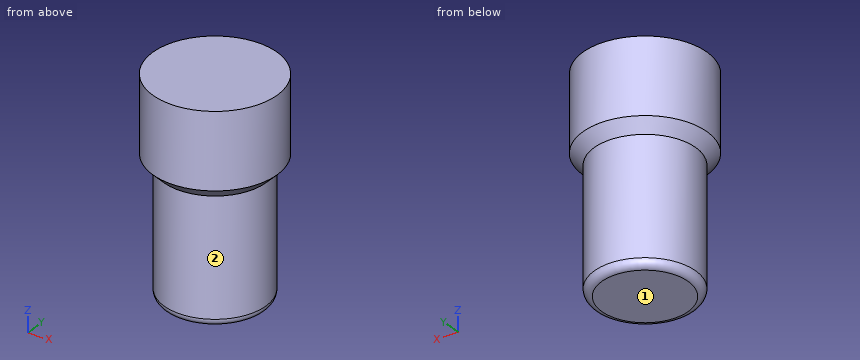
Autodesk Inventor part; units mm, degrees
ref_plane "YZ Plane" through (0, 0, 0) normal (1, 0, 0) x (0, 1, 0)
ref_plane "XZ Plane" through (0, 0, 0) normal (0, 1, 0) x (-1, 0, 0)
ref_plane "XY Plane" through (0, 0, 0) normal (0, 0, 1) x (1, 0, 0)
sketch "Sketch1" plane through (0, 0, 0) normal (0, 0, 1) x (1, 0, 0)
  circle A0 centre (0, 0) radius 13.5
  dimension "d0" = 27
extrude "Extrusion1" add sketch "Sketch1" along normal blind 36
sketch "Sketch2" plane through (0, 0, 36) normal (0, 0, 1) x (1, 0, 0)
  circle A0 centre (0, 0) radius 16.5
  dimension "d3" = 33
extrude "Extrusion2" add sketch "Sketch2" along normal blind 20
fillet "Fillet1" radius 2 1 edges at (-13.5, 0, 0)
chamfer "Chamfer1" distance 3 angle 45 1 edges at (-13.5, 0, 36)
properties part number "DispenserHead"
Part model, mm, in its own coordinate system. Face numbers are marked on the shaded views. A direction names the side the tool comes from. Round coordinates to 2 decimals unless told otherwise and drop trailing zeros. Write each loop counter-clockwise with the first axis right and the second up, starting at its lowest first coordinate (ties: lowest second). Pieces come first, ordered by that corner, then holes. Notation, with made-up numbers: M 55.25,-5 L 92.25,-5 A32 cw 92.25,26 Z; hole C 69,74.25 d6. An arc over 180 degrees is marked long. Answer as CSV lines item,"result". Start each with the question number.
1) Drill centre lines: L1, parallel to Y at x = 0, z = 19; L2, parallel to X at y = -0.5, z = 52.5; L3, parallel to Z at x = -10.5, y = -5. Where is each one in solid material? Low to high.
2) Drop flat-ended pins along their axis: pin 1 (2 mm diameter, centred on x = 3.5, z = 20.5, fed in from +Y); pin 2 (6 mm diameter, centred on y = -12, z = 15.5, fed in from +X); pin 3 (1.5 mm diameter, centred on y = -5.5, z = 36.5, fed in from -X). Give the stop position or say it passes through.
3) Band-saw the part on D-D (z = 46). List the corners of the cut face in (x, y), then the cut area to 3 significant figures.
4) Which spindle directions (+Z, -Z, +X, -X, +Y, -Y) get a long thin tool onto all of the face, cutting with end or side? Do the marked faces 1 and 2. Say none if no direction does.
5) Band-saw the part on C-C (z = 31). List the corners of the cut face in (x, y).
Worked out:
1,L1,"-13.5 to 13.5"
1,L2,"-16.49 to 16.49"
1,L3,"0 to 56"
2,pin 1,"y = 13.27"
2,pin 2,"x = 10.06"
2,pin 3,"x = -15.8"
3,outline,"C 0,0 d33"
3,area,"855 mm²"
4,face 1,"-Z, +X, -X, +Y, -Y"
4,face 2,"-Z"
5,outline,"C 0,0 d27"
